Part print with two shaded views. Sizes in mm from the minimum x, y, z corner. A direction names the side the tool comes from. Round coordinates to 2 decimals unless told otherwise and drop trailing zeros. Write each loop counter-clockwise with the first axis right and the second up, starting at its lowest first coordinate (ties: lowest second). Pieces come first, ordered by that corner, then holes. Notation, with made-up numbers: (32.25, 76.25) -> (60.25, 76.25) arc R19 ccw to (60.25, 103.25) -> close; hole circle Ø4 at (-23.5, 26). An arc over 180 degrees is marked (long way). Put each result on its own line as item: value. Start each with the question number.
1. Flat gauge pin, fed straight in: P1, Ø1, axis at x = 11.5, z = 7.5, coming from the -Y side. Where does the tip first touch, or does it go through?
2. Saw through at A-A on z = 10. List the corners of the cut face in (x, y), and give its area (3 significant figures).
3. Saw through at B-B on y = 5.25. List the corners of the cut face in (x, z).
4. Saw through at C-C on x = 21.75. List the corners of the cut face in (y, z).
5. Saw through at D-D on z = 12.5. List the corners of the cut face in (x, y) (1 decimal).
6. Drill centre lines: line 1 (X direction, y = 7.65, z = 10); line 2 (X direction, y = 4.5, z = 10); line 3 (Y direction, x = 16.75, z = 3). Where is each one in solid material? Low to high. Write a range as from..to.
7. 3-axis set-ups, long thin cutter, end or side, ignore diameter. For the marked faces 1 and 2: which of +Z, -Z, +X, -X, +Y, -Y reach the whole face in a straight line?
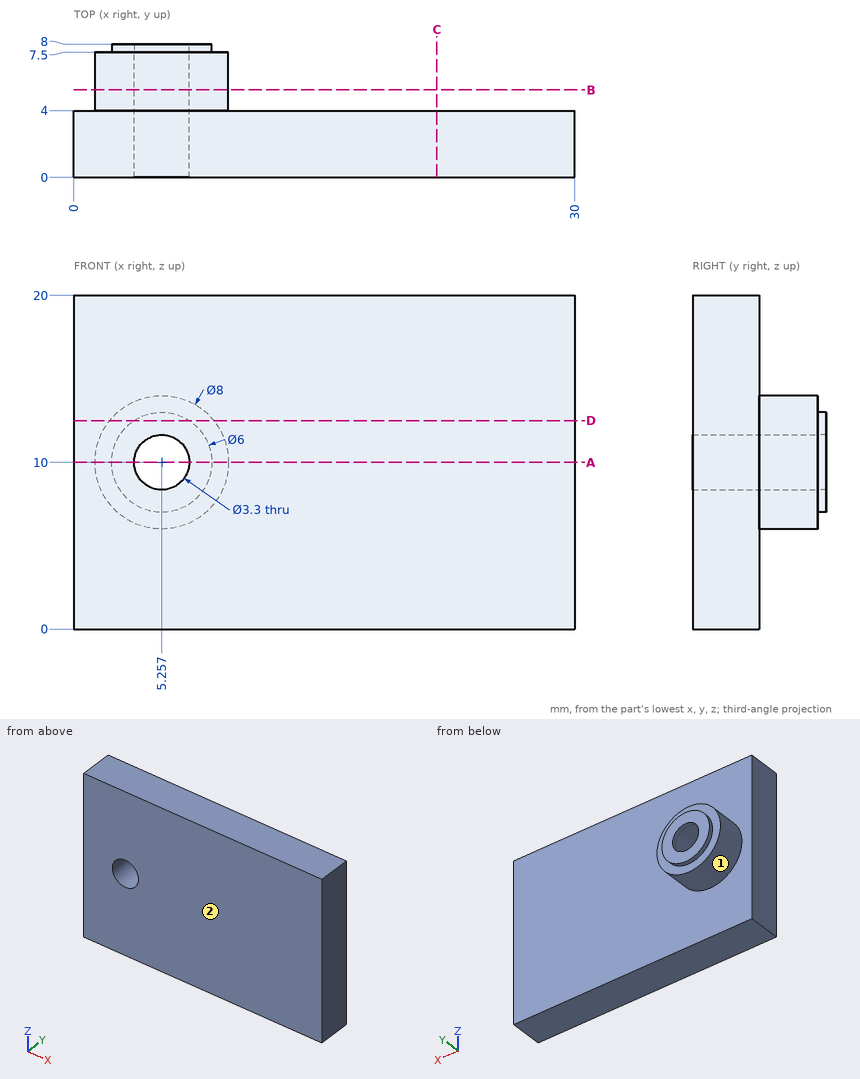
Return value:
1. P1: stops at y = 0
2. outline: (0, 0) -> (3.61, 0) -> (3.61, 8) -> (2.26, 8) -> (2.26, 7.5) -> (1.26, 7.5) -> (1.26, 4) -> (0, 4) -> close; (6.91, 0) -> (30, 0) -> (30, 4) -> (9.26, 4) -> (9.26, 7.5) -> (8.26, 7.5) -> (8.26, 8) -> (6.91, 8) -> close
2. area: 125 mm^2
3. outline: circle Ø8 at (5.26, 10); hole circle Ø3.3 at (5.26, 10)
4. outline: (0, 0) -> (4, 0) -> (4, 20) -> (0, 20) -> close
5. outline: (0, 0) -> (30, 0) -> (30, 4) -> (8.4, 4) -> (8.4, 7.5) -> (6.9, 7.5) -> (6.9, 8) -> (3.6, 8) -> (3.6, 7.5) -> (2.1, 7.5) -> (2.1, 4) -> (0, 4) -> close
6. line 1: x = 2.26..3.61, 6.91..8.26
6. line 2: x = 1.26..3.61, 6.91..9.26
6. line 3: y = 0..4
7. face 1: +Y
7. face 2: +Z, -Z, +X, -X, -Y
